The listing builds one solid part. Answer for the finished solid, in the listing's coordinates (mm). Face numbers are marked on the shaded views. A direction names the side the tool comes from. Coordinates: 2 decimals unless noted, no trailing zeros. Order: outer loops, then holes, each group sorted by start corner. A loop starts at its lowest first (then second) coordinate and runs counter-clockwise, first axis right, second up. Notation, with made-up numbers: (-17, -18.5) -> (25, -18.5) arc R25 cw to (25, 1.5) -> close; hole circle Ø8 at (0.5, 65.5). An arc over 180 degrees is marked (long way). Answer in a Markdown table with one row per item. Add a question column.
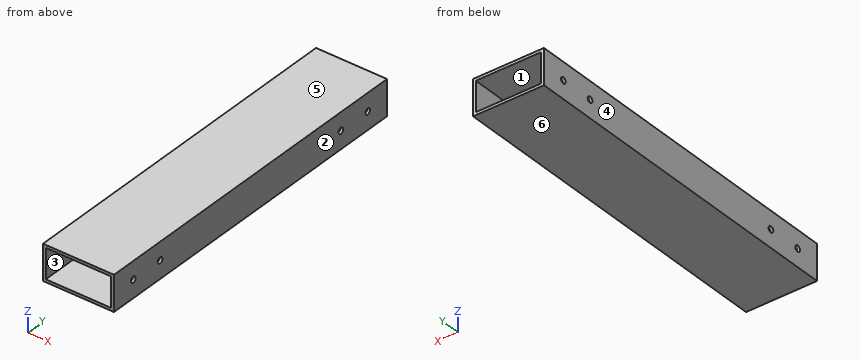
```python
from build123d import *

# Parameters (mm, degrees)
SKETCH_5_W          = 50.8
SKETCH_5_H          = 25.4
EXTRUDE_3_DEPTH     = 250
SKETCH_5_7_W        = 46.8
SKETCH_5_7_H        = 21.4
CUT_EXTRUDE_3_DEPTH = 252.607730406
SKETCH_6_R          = 2.150000004
SKETCH_6_R_2        = 2.15
CUT_EXTRUDE_4_DEPTH = 50.8


with BuildPart() as part:
    # 草圖5 → 填料-伸長3 (new body)
    with BuildSketch(Plane(origin=(0, 0, 0), x_dir=(1, 0, 0), z_dir=(0, 1, 0))):
        Rectangle(SKETCH_5_W, SKETCH_5_H)
    extrude(amount=EXTRUDE_3_DEPTH)

    # 草圖5<7> → 除料-伸長3 (cut, through all)
    with BuildSketch(Plane(origin=(0, 0, 0), x_dir=(1, 0, 0), z_dir=(0, 1, 0))):
        Rectangle(SKETCH_5_7_W, SKETCH_5_7_H)
    extrude(amount=CUT_EXTRUDE_3_DEPTH, mode=Mode.SUBTRACT)

    # 草圖6 → 除料-伸長4 (cut)
    with BuildSketch(Plane.ZY.offset(25.4)):
        with Locations((0, 232.300000014)):
            Circle(SKETCH_6_R)
        with Locations((0, 207.800000014)):
            Circle(SKETCH_6_R)
        with Locations((0, 42.2)):
            Circle(SKETCH_6_R_2)
        with Locations((0, 17.7)):
            Circle(SKETCH_6_R_2)
    extrude(amount=-CUT_EXTRUDE_4_DEPTH, mode=Mode.SUBTRACT)


solid = part.part
```
Q1. A cutting plane is placed at D-D (y = 226). Determine the outline of the cut face in (x, z), then the cut area to 3 significant figures.
Q2. A cutting plane is placed at C-C (z = 5). Determine the outline of the cut face in (x, y), then the cut area to 3 significant figures.
Q3. Given pin 1 (3.5 mm diameter, centred on y = 42.2, z = 0, fed in from -X); pin 2 (7 mm diameter, centred on y = 232.3, z = 0, fed in from -X), each flat-ended and moving along its own axis, determine where each tip first touches the part or whether it passes through.
Q4. A cutting plane is placed at A-A (x = -9). Determine the outline of the cut face in (y, z).
Q5. Determine the mould class of the marked faces 3, 4, 5 and 6 for opening direction Z: +Z half, -Z half, draft (parallel to the pull), parting line (faces both ways), or undercut.
Q6. Straight lines are drawn through the part: line 1 (Y direction, x = -24.8, z = 0); line 2 (X direction, y = 89.5, z = 3); line 3 (Z direction, x = -21, y = 236.5). For each, find the intervals that lie inside material, in ascending order.
Q7. For the marked faces 1 and 2, determine the directions among +Z, -Z, +X, -X, +Y, -Y from which every point of the face is accessible in a straight line to the end or side of a thin tool.
Q8. A cutting plane is placed at B-B (y = 42.2). Determine the outline of the cut face in (x, z).
Returned:
| question | item | result |
|---|---|---|
| 1 | outline | (-25.4, -12.7) -> (25.4, -12.7) -> (25.4, 12.7) -> (-25.4, 12.7) -> close; hole (-23.4, -10.7) -> (23.4, -10.7) -> (23.4, 10.7) -> (-23.4, 10.7) -> close |
| 1 | area | 289 mm² |
| 2 | outline | (-25.4, 0) -> (-23.4, 0) -> (-23.4, 250) -> (-25.4, 250) -> close; (23.4, 0) -> (25.4, 0) -> (25.4, 250) -> (23.4, 250) -> close |
| 2 | area | 1,000 mm² |
| 3 | pin 1 | passes through |
| 3 | pin 2 | stops at x = -25.4 |
| 4 | outline | (0, -12.7) -> (250, -12.7) -> (250, -10.7) -> (0, -10.7) -> close; (0, 10.7) -> (250, 10.7) -> (250, 12.7) -> (0, 12.7) -> close |
| 5 | face 3 | undercut |
| 5 | face 4 | draft |
| 5 | face 5 | +Z half |
| 5 | face 6 | -Z half |
| 6 | line 1 | y = 0 to 15.55, 19.85 to 40.05, 44.35 to 205.65, 209.95 to 230.15, 234.45 to 250 |
| 6 | line 2 | x = -25.4 to -23.4, 23.4 to 25.4 |
| 6 | line 3 | z = -12.7 to -10.7, 10.7 to 12.7 |
| 7 | face 1 | +Y, -Y |
| 7 | face 2 | +Z, -Z, +X, +Y, -Y |
| 8 | outline | (-25.4, -12.7) -> (25.4, -12.7) -> (25.4, -2.15) -> (23.4, -2.15) -> (23.4, -10.7) -> (-23.4, -10.7) -> (-23.4, -2.15) -> (-25.4, -2.15) -> close; (-25.4, 2.15) -> (-23.4, 2.15) -> (-23.4, 10.7) -> (23.4, 10.7) -> (23.4, 2.15) -> (25.4, 2.15) -> (25.4, 12.7) -> (-25.4, 12.7) -> close |
